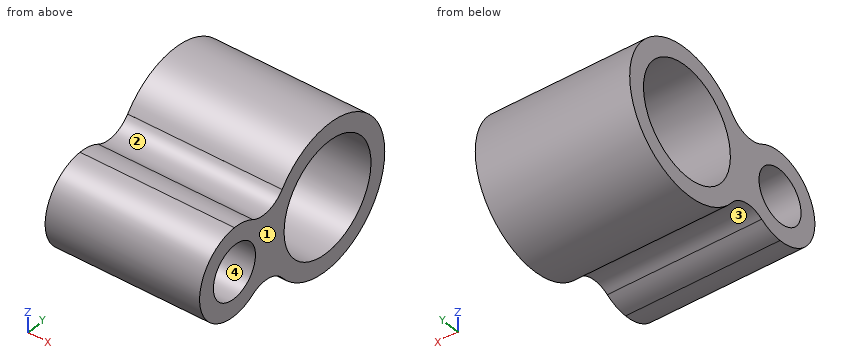
from build123d import *

# Parameters (mm, degrees)
SKETCH_1_R               = 12.6
SKETCH_1_R_2             = 6.1
EXTRUDE_1_DEPTH          = 35
CUT_EXTRUDE_1_DEPTH      = 54.637393673
CUT_EXTRUDE_1_DEPTH_BACK = 54.637393673


with BuildPart() as part:
    # 草图1 → 凸台-拉伸1 (new body)
    with BuildSketch(Plane(origin=(0, 0, 0), x_dir=(0, 0, -1), z_dir=(1, 0, 0))):
        with BuildLine():
            Line((-10.1, -27), (-10.1, -13.17383771))
            ThreePointArc((-10.1, -13.17383771), (0, 16.6), (10.1, -13.17383771))
            Line((10.1, -13.17383771), (10.1, -27))
            ThreePointArc((10.1, -27), (0, -37.1), (-10.1, -27))
        make_face()
        Circle(SKETCH_1_R, mode=Mode.SUBTRACT)
        with Locations((0, -27)):
            Circle(SKETCH_1_R_2, mode=Mode.SUBTRACT)
    extrude(amount=EXTRUDE_1_DEPTH)

    # 草图3 → 切除-拉伸1 (cut, two sides: drawn at the far end of the back side and taken through both)
    with BuildSketch(Plane(origin=(35, 0, 0), x_dir=(0, 0, -1), z_dir=(1, 0, 0)).offset(-CUT_EXTRUDE_1_DEPTH_BACK)):
        with BuildLine():
            Line((-16.628183068, -24.289618904), (-10.1, -27))
            ThreePointArc((-10.1, -27), (-9.71664565, -24.243771181), (-8.595683702, -21.696772521))
            ThreePointArc((-8.595683702, -21.696772521), (-16.131989791, -12.088249305), (-16.628183068, -24.289618904))
        make_face()
        with BuildLine():
            Line((10.1, -27), (14.395468751, -24.781680805))
            ThreePointArc((14.395468751, -24.781680805), (17.188775236, -12.535721906), (8.595683702, -21.696772521))
            ThreePointArc((8.595683702, -21.696772521), (9.71664565, -24.243771181), (10.1, -27))
        make_face()
    extrude(amount=CUT_EXTRUDE_1_DEPTH + CUT_EXTRUDE_1_DEPTH_BACK, mode=Mode.SUBTRACT)


solid = part.part
Verification items for the finished model (mm, model axes). Face numbers are marked on the shaded views. Give positions to 0.01 mm unless a question says otherwise; leave off trailing zeros. Write each loop counter-clockwise with the first axis right and the second up, starting at its lowest first coordinate (ties: lowest second). Pieces come first, ordered by that corner, then holes. Notation, with made-up numbers: M -37,9 L -11,9 A11 cw -11,28 Z; hole C 89.5,45 d6. An arc over 180 degrees is marked long. Put each result on its own line as item: value. Start each with the question number.
1. Section check B-B (y = 0). Record the cut outline in (x, z).
2. Section check A-A (x = 17). Give the number of separate pieces and of enclosed holes in the cut face, and give its area (3 significant figures).
3. Scan lines: line 1 along Y through (x, z) = (11, 0); line 2 along Y through (x, z) = (3, 3.5); line 3 along Y through (x, z) = (22.5, -7.5). Record each from-to range of solid material in increasing order. Write a range as [from, to].
4. Draft check along Z on the marked faces 1, 2, 3 and 4. Enter one of: +Z half, -Z half, draft (parallel to the pull), parting line (faces both ways), or undercut.
5. Section check C-C (z = 0). Record the cut outline in (x, y).
6. Go/stop test with flat-tipped pins: pin 1 Ø5 at (x, y) = (13, -30) entering from -Z; pin 2 Ø2 at (x, y) = (28, -24) entering from +Z; pin 3 Ø7.5 at (y, z) = (-27, 0) entering from -X; pin 4 Ø4 at (x, y) = (31, -19) entering from -Z. Record where each tip stops, or that it passes through.
7. Section check D-D (z = -3.5). Record the cut outline in (x, y).
Answer list:
1. outline: M 0,-16.6 L 35,-16.6 L 35,-12.6 L 0,-12.6 Z; M 0,12.6 L 35,12.6 L 35,16.6 L 0,16.6 Z
2. separate pieces: 1
2. enclosed holes: 2
2. area: 605 mm2
3. line 1: [-37.1, -33.1], [-20.9, -12.6], [12.6, 16.6]
3. line 2: [-36.47, -32], [-22, -12.1], [12.1, 16.23]
3. line 3: [-33.76, -10.12], [10.12, 14.81]
4. face 1: draft
4. face 2: +Z half
4. face 3: -Z half
4. face 4: undercut
5. outline: M 0,-37.1 L 35,-37.1 L 35,-33.1 L 0,-33.1 Z; M 0,-20.9 L 35,-20.9 L 35,-12.6 L 0,-12.6 Z; M 0,12.6 L 35,12.6 L 35,16.6 L 0,16.6 Z
6. pin 1: z = -10.09
6. pin 2: z = 9.9
6. pin 3: through
6. pin 4: z = -8.22
7. outline: M 0,-36.47 L 35,-36.47 L 35,-32 L 0,-32 Z; M 0,-22 L 35,-22 L 35,-12.1 L 0,-12.1 Z; M 0,12.1 L 35,12.1 L 35,16.23 L 0,16.23 Z
